Check sheet for the modelled part. Datum: model origin and axes. Units: mm. A direction names the side the tool comes from. Give positions to 0.01 mm unless a question says otherwise; leave off trailing zeros. Write each loop counter-clockwise with the first axis right and the second up, starting at its lowest first coordinate (ties: lowest second). Pieces come first, ordered by that corner, then holes. Notation, with made-up numbers: (-28.5, -8) -> (-11.5, -8) arc R35 cw to (-11.5, 27) -> close; hole circle Ø5 at (-31, -2.75). An arc over 180 degrees is marked (long way). Use a Markdown table: item, result. Add a question column.
1. Release check for a two-part mould opening along Y. For faces 6 (the flat face through (40, 0, 3)), 7 (the flat face through (30, 10, 0)), 8 (the flat face through (0.485, 9.895, 2.769)), 9 (the flat face through (20.75, 20.65, 2.69)) record: released by +Y, released by -Y, zero draft, split by the parting line, or undercut.
2. Cross-section at D-D (y = 2.75). Enter the section's corners in (x, z).
3. Cross-section at B-B (z = 1.8). Enter the section's corners in (x, y) (3 decimals).
4. Cross-section at A-A (y = 20). Enter the section's corners in (x, z), then the cut area to 3 significant figures.
5. Gauge pin test, flat end, axial feed: P1, Ø3, axis at x = 69.5, z = 1.5, coming from the +Y side. Record the tip position at first contact, or that the pin passes through.
6. Cross-section at C-C (x = 33.5). Enter the section's corners in (y, z), then the cut area to 3 significant figures.
7. Set-up check for faces 1 (the flat face through (57.474, 10.829, 2.769)), 2 (the flat face through (1.573, 4.559, 2.692)), 3 (the flat face through (0.04, 16.86, 2.77)), 4 (the flat face through (4.699, 21.876, 2.769)), 5 (the flat face through (30, 10, 5.461)): record each of +Z, -Z, +X, -X, +Y, -Y from which the full face is reachable in a straight line by a thin tool's end or side.
8. Scan lines: probe 1 along Y at (x, z) = (35, 1.45); probe 2 along Y at (x, z) = (4.5, 0.75); probe 3 along X at (y, z) = (11.5, 1.9). Record each from-to range of solid material in increasing order. Write a range as [from, to].
from build123d import *

# Parameters (mm, degrees)
BOSS_EXTRUDE1_DEPTH = 5.461
BOSS_EXTRUDE2_DEPTH = 5.461


with BuildPart() as part:
    # Sketch1 → Boss-Extrude1 (new body)
    with BuildSketch(Plane.XY):
        Polygon((0, 0), (80.607391231, 0), (8.573798388, 24.851589531), align=None)
    extrude(amount=BOSS_EXTRUDE1_DEPTH)

    # Sketch2 → Boss-Extrude2 (add)
    with BuildSketch(Plane.XY.offset(5.461)):
        Polygon((7.244238348, 20.997792314), (2.081830861, 22.778822897), (-2.060100727, 10.77322409), (3.10230676, 8.992193507), align=None)
        Polygon((32.584996002, 16.567726354), (56.596193616, 8.283863177), (58.377224199, 13.446270664), (34.366026585, 21.730133841), align=None)
    extrude(amount=-BOSS_EXTRUDE2_DEPTH)


solid = part.part
Worked answers:
| question | item | result |
|---|---|---|
| 1 | face 6 | released by -Y |
| 1 | face 7 | zero draft |
| 1 | face 8 | undercut |
| 1 | face 9 | released by +Y |
| 2 | outline | (0.95, 0) -> (72.64, 0) -> (72.64, 5.46) -> (0.95, 5.46) -> close |
| 3 | outline | (-2.06, 10.773) -> (3.102, 8.992) -> (0, 0) -> (80.607, 0) -> (56.596, 8.284) -> (58.377, 13.446) -> (34.366, 21.73) -> (32.585, 16.568) -> (8.574, 24.852) -> (7.244, 20.998) -> (2.082, 22.779) -> close |
| 4 | outline | (1.12, 0) -> (22.64, 0) -> (22.64, 5.46) -> (1.12, 5.46) -> close; (33.77, 0) -> (39.38, 0) -> (39.38, 5.46) -> (33.77, 5.46) -> close |
| 4 | area | 148 mm² |
| 5 | P1 | stops at y = 4.35 |
| 6 | outline | (0, 0) -> (19.22, 0) -> (19.22, 5.46) -> (0, 5.46) -> close |
| 6 | area | 105 mm² |
| 7 | face 1 | +Z, -Z, +X |
| 7 | face 2 | +Z, -Z, -X |
| 7 | face 3 | +Z, -Z, -X, +Y |
| 7 | face 4 | +Z, -Z, +Y |
| 7 | face 5 | +Z, +X, -X, +Y, -Y |
| 8 | probe 1 | y = [0, 21.51] |
| 8 | probe 2 | y = [0, 21.94] |
| 8 | probe 3 | x = [-1.81, 57.71] |
